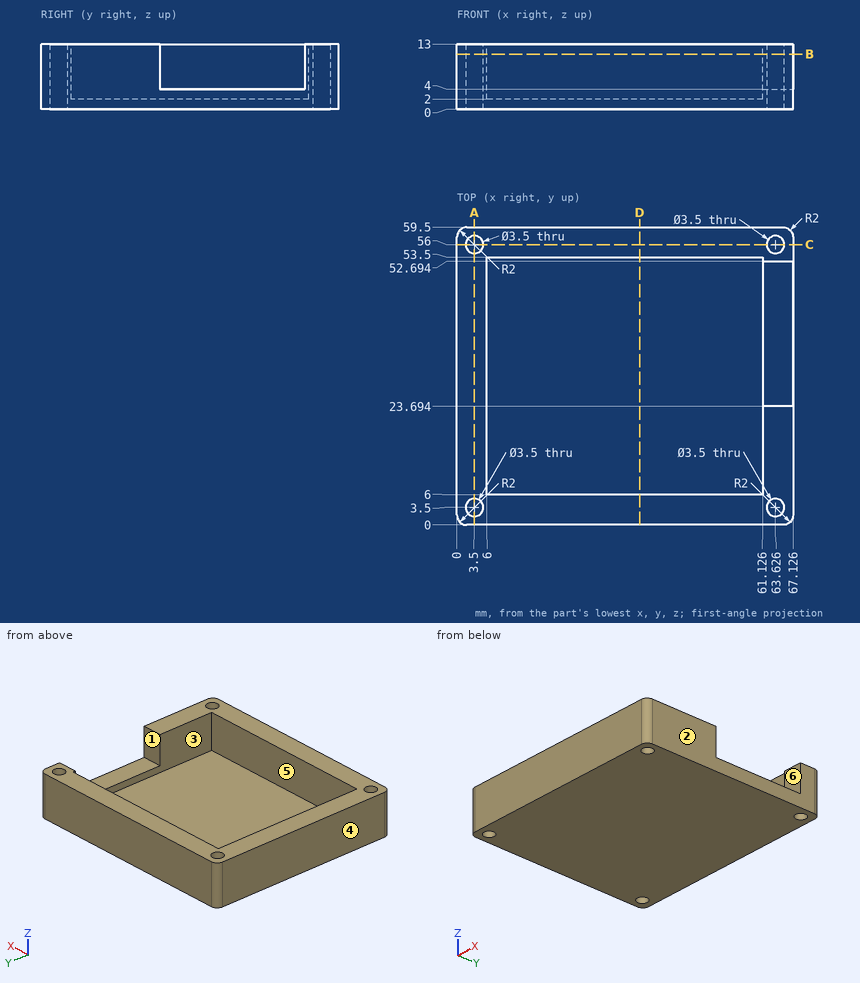
Drawing for the job (mm, zero at the part's lowest x, y, z). A direction names the side the tool comes from. Coordinates: 2 decimals unless noted, no trailing zeros. Order: outer loops, then holes, each group sorted by start corner. A loop starts at its lowest first (then second) coordinate and runs counter-clockwise, first axis right, second up. Notation, with made-up numbers: (86.5, 83) - (126.5, 83) arc R16 ccw to (126.5, 112) - close; hole circle Ø3 at (35, 45.25). An arc over 180 degrees is marked (long way). Use a Markdown table: item, result. Add a question column.
(1) Saw through at A-A (x = 3.5). Give the cut face in (y, z).
(2) Pull direction X, two halves, no side cores. Call the marked faces 1, 2 and 3: +X half, -X half, draft (parallel to the pull), parting line (faces both ways), or undercut.
(3) Which spindle directions (+Z, -Z, +X, -X, +Y, -Y) get a long thin tool onto all of the face, cutting with end or side? Do the marked faces 4, 5 and 6. Say none if no direction does.
(4) Saw through at B-B (z = 11). Give the cut face in (x, y).
(5) Flat gauge pins, fed straight in: pin 1 (10 mm diameter, centred on x = 16.5, y = 29, fed in from +Z); pin 2 (3 mm diameter, centred on x = 65, y = 39, fed in from +Z); pin 3 (3 mm diameter, centred on x = 63.626, y = 3.5, fed in from -Z). Where does each tip first touch, or does it go through?
(6) Saw through at C-C (y = 56). Give the cut face in (x, z), then the cut area to 3 significant figures.
(7) Drill centre lines: line 1 along Y through (x, z) = (3.5, 5.25); line 2 along Y through (x, z) = (13.5, 4.5); line 3 along X through (y, z) = (5, 7.25) (1 decimal). Where is each one in solid material? Low to high. Write a range as [from, to].
(8) Saw through at D-D (x = 36.5). Give the cut face in (y, z), then the cut area to 3 significant figures.
Solved:
| question | item | result |
|---|---|---|
| 1 | outline | (0, 0) - (1.75, 0) - (1.75, 13) - (0, 13) - close; (5.25, 0) - (54.25, 0) - (54.25, 13) - (5.25, 13) - close; (57.75, 0) - (59.5, 0) - (59.5, 13) - (57.75, 13) - close |
| 2 | face 1 | draft |
| 2 | face 2 | +X half |
| 2 | face 3 | undercut |
| 3 | face 4 | +Z, -Z, -X, +Y, -Y |
| 3 | face 5 | +Z |
| 3 | face 6 | +Z, +X |
| 4 | outline | (0, 2) arc R2 ccw to (2, 0) - (65.13, 0) arc R2 ccw to (67.13, 2) - (67.13, 23.69) - (61.13, 23.69) - (61.13, 6) - (6, 6) - (6, 53.5) - (61.13, 53.5) - (61.13, 52.69) - (67.13, 52.69) - (67.13, 57.5) arc R2 ccw to (65.13, 59.5) - (2, 59.5) arc R2 ccw to (0, 57.5) - close; hole circle Ø3.5 at (3.5, 3.5); hole circle Ø3.5 at (3.5, 56); hole circle Ø3.5 at (63.63, 3.5); hole circle Ø3.5 at (63.63, 56) |
| 5 | pin 1 | stops at z = 2 |
| 5 | pin 2 | stops at z = 4 |
| 5 | pin 3 | passes through |
| 6 | outline | (0, 0) - (1.75, 0) - (1.75, 13) - (0, 13) - close; (5.25, 0) - (61.88, 0) - (61.88, 13) - (5.25, 13) - close; (65.38, 0) - (67.13, 0) - (67.13, 13) - (65.38, 13) - close |
| 6 | area | 782 mm² |
| 7 | line 1 | y = [0, 1.75], [5.25, 54.25], [57.75, 59.5] |
| 7 | line 2 | y = [0, 6], [53.5, 59.5] |
| 7 | line 3 | x = [0, 2.6], [4.4, 62.7], [64.5, 67.1] |
| 8 | outline | (0, 0) - (59.5, 0) - (59.5, 13) - (53.5, 13) - (53.5, 2) - (6, 2) - (6, 13) - (0, 13) - close |
| 8 | area | 251 mm² |
